The figure shows three views and two pictorial views of one solid part (mm, origin at its lowest corner). Answer the questions. Coordinates: 2 decimals unless noted, no trailing zeros. Write each loop counter-clockwise with the first axis right and the second up, starting at its lowest first coordinate (ties: lowest second). Pieces come first, ordered by that corner, then holes. Notation, with made-up numbers: M 26.5,30 L 34.5,30 A19 ccw 34.5,47 Z; hole C -15,10.5 d6. An arc over 180 degrees is marked long. Write item = value, one per line.
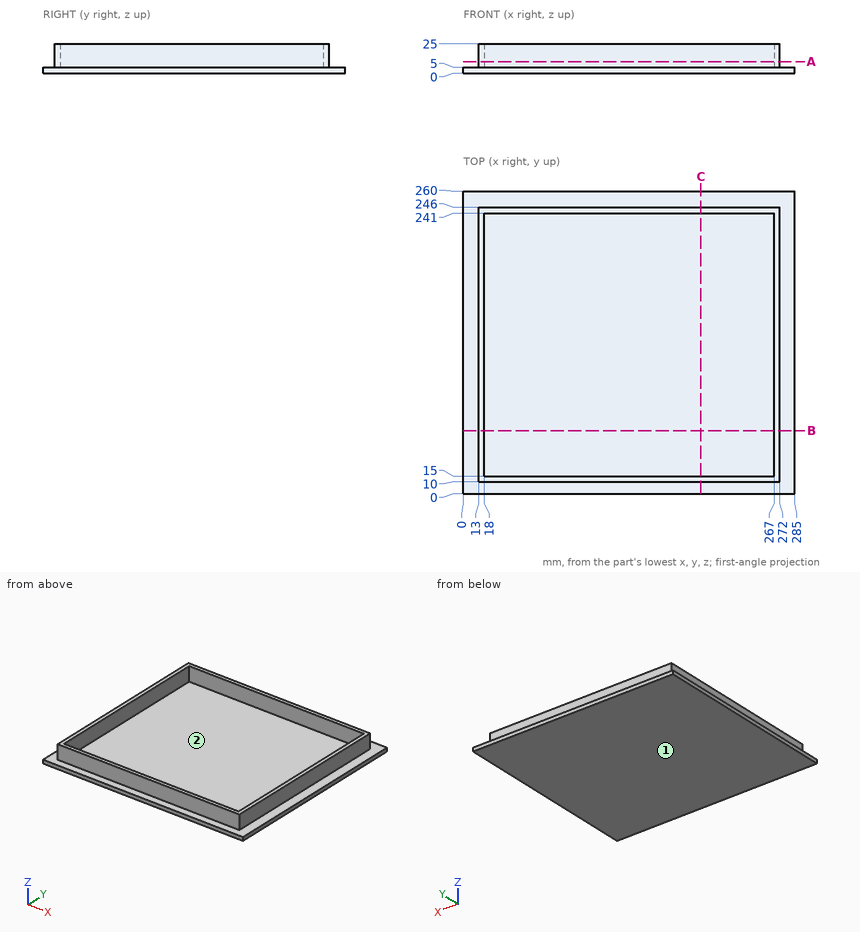
Item 1: Find section C-C (x = 204). Determine the outline of the cut face in (y, z).
Worked answers:
outline = M 0,0 L 260,0 L 260,5 L 246,5 L 246,25 L 241,25 L 241,5 L 15,5 L 15,25 L 10,25 L 10,5 L 0,5 Z
Item 2: Consider line 1 along Y through (x, z) = (89, 5.75); line 2 along X through (y, z) = (19, 20.75); line 3 along Z through (x, y) = (250, 149). Determine where each line is inside the solid, lowest interval first. Write a range as from..to.
Worked answers:
line_1 = 10..15, 241..246
line_2 = 13..18, 267..272
line_3 = 0..5
Item 3: Find section A-A (z = 9.75). Determine the outline of the cut face in (x, y), and give its area (3 significant figures).
Worked answers:
outline = M 13,10 L 272,10 L 272,246 L 13,246 Z; hole M 18,15 L 267,15 L 267,241 L 18,241 Z
area = 4,850 mm²
Item 4: Flat-ended cylindrical pins translate along their axes: pin 1 (3 mm diameter, centred on x = 132, y = 178, fed in from -Z); pin 2 (3 mm diameter, centred on x = 66.5, y = 155, fed in from +Z); pin 3 (10 mm diameter, centred on y = 84, z = 16.5, fed in from -X); pin 4 (6 mm diameter, centred on y = 200, z = 18, fed in from +X). Find the tip coordinate at first contact, or state that the pin passes through.
Worked answers:
pin_1 = 0
pin_2 = 5
pin_3 = 13
pin_4 = 272
Item 5: For a pull along X with two mould halves and no side action, classify the marked faces 1 and 2 as released by +X, released by -X, zero draft, split by the parting line, or undercut.
Worked answers:
face_1 = zero draft
face_2 = undercut
Item 6: Find section B-B (y = 54). Determine the outline of the cut face in (x, z), and give its area (4 significant figures).
Worked answers:
outline = M 0,0 L 285,0 L 285,5 L 272,5 L 272,25 L 267,25 L 267,5 L 18,5 L 18,25 L 13,25 L 13,5 L 0,5 Z
area = 1,625 mm²
